The listing builds one solid part. Answer for the finished solid, in the listing's coordinates (mm). Face numbers are marked on the shaded views. A direction names the side the tool comes from. Round coordinates to 2 decimals unless told otherwise and drop trailing zeros. Write each loop counter-clockwise with the first axis right and the second up, starting at its lowest first coordinate (ties: lowest second). Pieces come first, ordered by that corner, then holes.
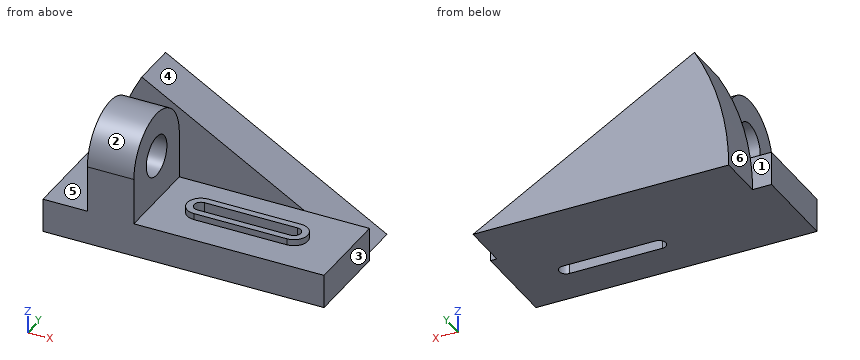
from build123d import *

# Parameters (mm, degrees)
F1_DEPTH  = 22
F2_W      = 133
F2_H      = 16
F3_DEPTH  = 42
F4_W      = 22
F4_H      = 42
F5_DEPTH  = 22
F7_DEPTH  = 22
F8_DEPTH  = 43.001
F10_DEPTH = 3
F11_DEPTH = 16.001


with BuildPart() as f1:
    # F0 (on Front) → F1 (new body)
    with BuildSketch(Plane.XZ):
        with BuildLine():
            ThreePointArc((16.210926, 60.5), (4.122975, 31.317104), (0, 0))
            Line((0, 0), (121, 0))
            Line((121, 0), (16.210926, 60.5))
        make_face()
    extrude(amount=-F1_DEPTH)

    # F2 (on Front) → F3 (join)
    with BuildSketch(Plane.XZ):
        with Locations((57.5, 8)):
            Rectangle(F2_W, F2_H)
    extrude(amount=F3_DEPTH)

    # F4 (on face) → F5 (join)
    with BuildSketch(Plane.XY.offset(16)):
        with Locations((23, -21)):
            Rectangle(F4_W, F4_H)
    extrude(amount=F5_DEPTH)

    # F6 (on face) → F7 (join, through all)
    with BuildSketch(Plane.YZ.offset(34)):
        with BuildLine():
            ThreePointArc((-30.5, 38), (-21, 47.5), (-11.5, 38))
            Line((-11.5, 38), (0, 38))
            ThreePointArc((0, 38), (-21, 59), (-42, 38))
            Line((-42, 38), (-30.5, 38))
        make_face()
    extrude(amount=-F7_DEPTH)

    # F6 (on face) → F8 (cut, through all)
    with BuildSketch(Plane.YZ.offset(34)):
        with BuildLine():
            ThreePointArc((-30.5, 38), (-21, 28.5), (-11.5, 38))
            Line((-11.5, 38), (-30.5, 38))
        make_face()
    extrude(amount=-F8_DEPTH, mode=Mode.SUBTRACT)

    # F9 (on face) → F10 (join)
    with BuildSketch(Plane.XY.offset(16)):
        with BuildLine():
            ThreePointArc((55, -14.5), (48.5, -21), (55, -27.5))
            Line((55, -27.5), (99, -27.5))
            ThreePointArc((99, -27.5), (105.5, -21), (99, -14.5))
            Line((99, -14.5), (55, -14.5))
        make_face()
        with BuildLine():
            Line((99, -24.25), (55, -24.25))
            ThreePointArc((55, -24.25), (51.75, -21), (55, -17.75))
            Line((55, -17.75), (99, -17.75))
            ThreePointArc((99, -17.75), (102.25, -21), (99, -24.25))
        make_face(mode=Mode.SUBTRACT)
    extrude(amount=F10_DEPTH)

    # F10_face (on face) → F11 (cut, through all)
    with BuildSketch(Plane(origin=(77, -21, 16), x_dir=(1, 0, 0), z_dir=(0, 0, 1))):
        with BuildLine():
            ThreePointArc((22, -3.25), (25.25, 0), (22, 3.25))
            Line((22, 3.25), (-22, 3.25))
            ThreePointArc((-22, 3.25), (-25.25, 0), (-22, -3.25))
            Line((-22, -3.25), (22, -3.25))
        make_face()
    extrude(amount=-F11_DEPTH, mode=Mode.SUBTRACT)


solid = f1.part
1. For a pull along Y with two mould halves and no side action, classify the marked faces 1, 2 and 3 as released by +Y, released by -Y, zero draft, split by the parting line, or undercut.
Geometry says:
face 1: released by +Y
face 2: undercut
face 3: zero draft
2. A tool of negligible diameter and unlimited length cuts with its end or side. For the marked faces 4, 5 and 6, from which of +Z, -Z, +X, -X, +Y, -Y can it reach the whole face along a straight path? Write none if from no direction.
Geometry says:
face 4: +Z, +X, +Y
face 5: +Z, -X, -Y
face 6: +Z, -X, +Y
3. Section C-C on x = 62.5 is taken. Determine the outline of the cut face in (y, z) (3 decimals).
Geometry says:
outline: (-42, 0) - (-24.25, 0) - (-24.25, 19) - (-27.5, 19) - (-27.5, 16) - (-42, 16) - close; (-17.75, 0) - (22, 0) - (22, 33.775) - (0, 33.775) - (0, 16) - (-14.5, 16) - (-14.5, 19) - (-17.75, 19) - close
4. Section A-A on y = -21 is taken. Determine the outline of the cut face in (x, z), plus the area to 3 significant figures.
Geometry says:
outline: (-9, 0) - (51.75, 0) - (51.75, 19) - (48.5, 19) - (48.5, 16) - (34, 16) - (34, 28.5) - (12, 28.5) - (12, 16) - (-9, 16) - close; (12, 47.5) - (34, 47.5) - (34, 59) - (12, 59) - close; (102.25, 0) - (124, 0) - (124, 16) - (105.5, 16) - (105.5, 19) - (102.25, 19) - close
area: 1,870 mm2
5. Given pin 1 (5 mm diameter, centred on y = -18, z = 30, fed in from -X); pin 2 (10 mm diameter, centred on x = 82.5, y = 2, fed in from +Z); pin 3 (4 mm diameter, centred on x = 64, y = -18, fed in from +Z), each flat-ended and moving along its own axis, determine where each tip first touches the part or whether it passes through.
Geometry says:
pin 1: stops at x = 12
pin 2: stops at z = 25.11
pin 3: stops at z = 19
6. Section B-B on z = 41 is taken. Determine the outline of the cut face in (x, y).
Geometry says:
outline: (7.16, 0) - (49.99, 0) - (49.99, 22) - (7.16, 22) - close; (12, -41.78) - (34, -41.78) - (34, -30.01) - (12, -30.01) - close; (12, -11.99) - (34, -11.99) - (34, -0.22) - (12, -0.22) - close
7. Section D-D on x = 104 is taken. Determine the outline of the cut face in (y, z).
Geometry says:
outline: (-42, 0) - (22, 0) - (22, 9.81) - (0, 9.81) - (0, 16) - (-16.85, 16) - (-16.85, 19) - (-25.15, 19) - (-25.15, 16) - (-42, 16) - close
8. Straight lines are drawn through the part: line 1 along Z through (x, y) = (22, -21); line 2 along Y through (x, z) = (85.5, 9); line 3 along X through (y, z) = (-18, 17). For each, find the intervals that lie inside material, in ascending order.
Geometry says:
line 1: z = 0 to 28.5, 47.5 to 59
line 2: y = -42 to -24.25, -17.75 to 22
line 3: x = 12 to 34, 49.23 to 53.75, 100.25 to 104.77
